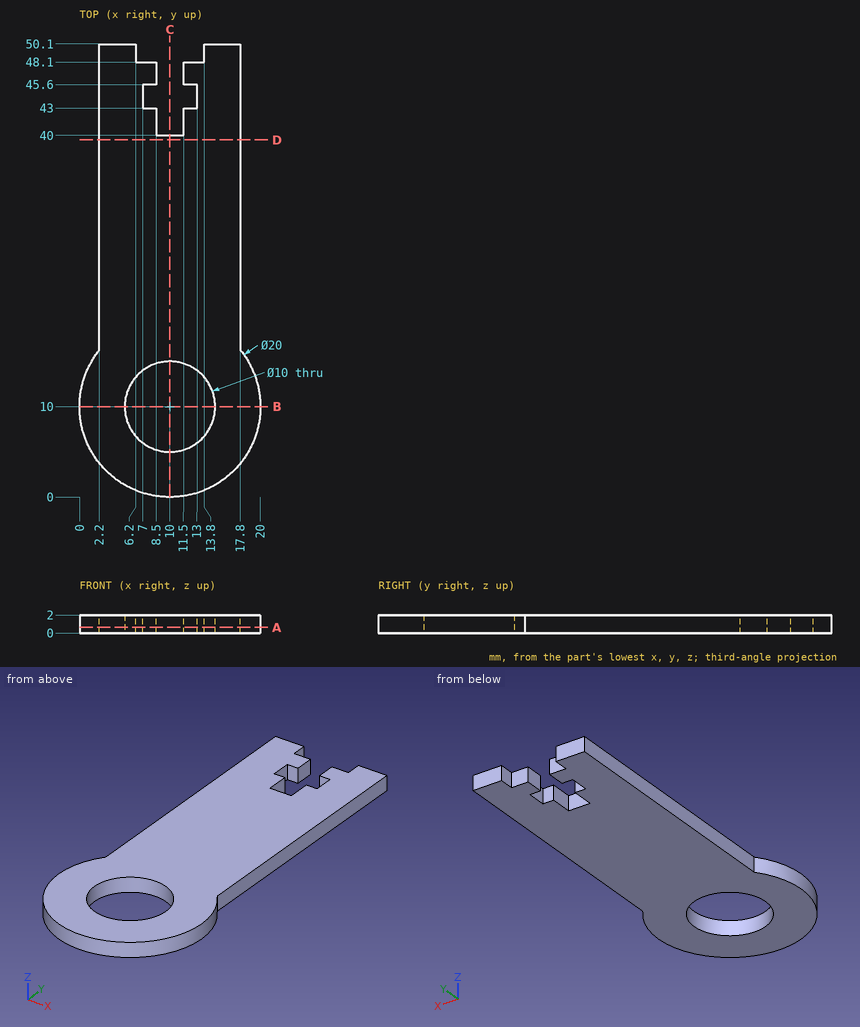
Verification items for this drawing (mm, ordinates from the low corner). Give positions to 0.01 mm unless a question says otherwise; leave off trailing zeros. Loops run counter-clockwise (first coordinate to the right, second up) from the corner with the lowest first, then second, coordinate; pieces in that order, holes last. Notation, with made-up numbers: M 43.5,84.5 L 54.5,84.5 A6 cw 54.5,92.5 Z; hole C 87.5,68 d10. An arc over 180 degrees is marked long. Answer as a JSON object with one key per item and string values. Group by question number.
Q1. Material ranges on line 1 along X through (y, z) = (40.5, 1.4); line 2 along X through (y, z) = (33.5, 1.8); line 3 along Y through (x, z) = (18.75, 0.55), recorded low to high. Write a range as [from, to].
Q2. Cross-section at C-C on x = 10. Record the cut outline in (y, z).
Q3. Cross-section at D-D on y = 39.5. Record the cut outline in (x, z).
Q4. Cross-section at A-A on z = 0.65. Record the cut outline in (x, y), then the cut area to 3 significant figures.
Q5. Go/stop test with flat-tipped pins: P1, Ø0.6, axis at y = 44.5, z = 0.5, coming from the +X side; P2, Ø0.6, axis at y = 49, z = 1, coming from the -X side; P3, Ø1, axis at x = 13, z = 1, coming from the +Y side. Record where each tip stops, or that it passes through.
Q6. Cross-section at B-B on y = 10. Record the cut outline in (x, z), then the cut area to 3 significant figures.
Evaluation:
{
 "1": {"line 1": "x = [2.2, 8.5], [11.5, 17.8]", "line 2": "x = [2.2, 17.8]", "line 3": "y = [5.16, 14.84]"},
 "2": {"outline": "M 0,0 L 5,0 L 5,2 L 0,2 Z; M 15,0 L 40,0 L 40,2 L 15,2 Z"},
 "3": {"outline": "M 2.2,0 L 17.8,0 L 17.8,2 L 2.2,2 Z"},
 "4": {"outline": "M 2.2,16.26 A10 ccw long 17.8,16.26 L 17.8,50.1 L 13.8,50.1 L 13.8,48.1 L 11.5,48.1 L 11.5,45.6 L 13,45.6 L 13,43 L 11.5,43 L 11.5,40 L 8.5,40 L 8.5,43 L 7,43 L 7,45.6 L 8.5,45.6 L 8.5,48.1 L 6.2,48.1 L 6.2,50.1 L 2.2,50.1 Z; hole C 10,10 d10", "area": "676 mm2"},
 "5": {"P1": "stops at x = 17.8", "P2": "stops at x = 2.2", "P3": "stops at y = 48.1"},
 "6": {"outline": "M 0,0 L 5,0 L 5,2 L 0,2 Z; M 15,0 L 20,0 L 20,2 L 15,2 Z", "area": "20.0 mm2"}
}
